from build123d import *

# Parameters (mm, degrees)
SKETCH1_W                         = 40
SKETCH1_H                         = 30
BOSS_EXTRUDE1_DEPTH               = 40
F_1_2_CLEARANCE_HOLE1_D           = 13.49248
F_1_2_CLEARANCE_HOLE1_CSINK_D     = 14.76248
F_1_2_CLEARANCE_HOLE1_CSINK_ANGLE = 100
CUT_EXTRUDE1_REACH                = 60.523
SKETCH4_R                         = 5
FILLET1_R                         = 5


with BuildPart() as part:
    # Sketch1 → Boss-Extrude1 (new body)
    with BuildSketch(Plane(origin=(0, 0, 0), x_dir=(1, 0, 0), z_dir=(0, 1, 0))):
        Rectangle(SKETCH1_W, SKETCH1_H)
    extrude(amount=BOSS_EXTRUDE1_DEPTH)

    # 1/2 Clearance Hole1 (through all)
    with Locations(Plane.XY.offset(15)):
        with Locations((0, 25)):
            CounterSinkHole(F_1_2_CLEARANCE_HOLE1_D / 2, F_1_2_CLEARANCE_HOLE1_CSINK_D / 2, counter_sink_angle=F_1_2_CLEARANCE_HOLE1_CSINK_ANGLE)

    # Sketch4 → Cut-Extrude1 (cut, up to next)
    with BuildSketch(Plane(origin=(20, 0, 0), x_dir=(0, 0, -1), z_dir=(1, 0, 0)), mode=Mode.PRIVATE) as cut_extrude1_sk1:
        with Locations((0, 10)):
            Circle(SKETCH4_R)
    cut_extrude1_tool1 = extrude(cut_extrude1_sk1.sketch, amount=-CUT_EXTRUDE1_REACH, mode=Mode.PRIVATE) & part.part
    add(cut_extrude1_tool1.solids().sort_by_distance((20, 10, 0))[0], mode=Mode.SUBTRACT)

    # Fillet1
    fillet1_edges = [part.edges().sort_by_distance(p)[0] for p in [
        (-20, 40, 0),
        (6.74624, 25, -15),
        (20, 40, 0),
        (-20, 0, 0),
        (20, 0, 0),
    ]]
    fillet(fillet1_edges, radius=FILLET1_R - 0.0001)  # a hair under: the kernel refuses the full size


solid = part.part
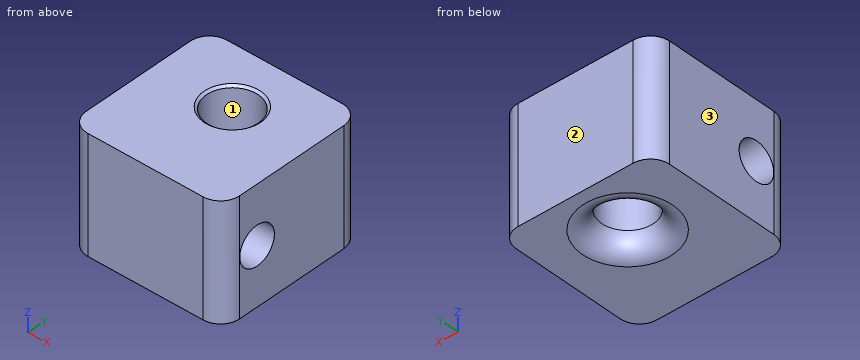
Check sheet for the modelled part. Datum: model origin and axes. Units: mm. Face numbers are marked on the shaded views. Round coordinates to 2 decimals unless told otherwise and drop trailing zeros. Loops run counter-clockwise (first coordinate to the right, second up) from the corner with the lowest first, then second, coordinate; pieces in that order, holes last.
1. Mould release check, pull along Y, two halves, no side actions. Record for the marked faces 1, 2 and 3: released by +Y, released by -Y, zero draft, split by the parting line, or undercut.
2. Gauge pin test, flat ends, axial feed: pin 1 Ø8 at (x, y) = (-3, 24) entering from -Z; pin 2 Ø12 at (x, y) = (0, 25) entering from +Z. Record the tip position at first contact, or that the pin passes through.
3. Sectioned sample at A-A on x = 0. Record the boundary of the cut face in (y, z).
4. Scan lines: probe 1 along Y at (x, z) = (-10, 0); probe 2 along X at (y, z) = (25, 7.75); probe 3 along Y at (x, z) = (1, -0.25). Record each from-to range of solid material in increasing order.
5. Sectioned sample at B-B on y = 25. Record the boundary of the cut face in (x, z), and give its area (3 significant figures).
6. Sectioned sample at C-C on z = 0. Give the number of separate pieces and of enclosed holes in the cut face, and give its area (3 significant figures).
7. Sectioned sample at D-D on z = -8. Record the boundary of the cut face in (x, y).
Recorded:
1. face 1: undercut
1. face 2: released by +Y
1. face 3: zero draft
2. pin 1: stops at z = -12
2. pin 2: passes through
3. outline: (0, -15) - (13.25, -15) arc R5 ccw to (18.25, -10) - (18.25, 14.47) - (17.62, 15) - (0, 15) - close; (31.75, -10) arc R5 ccw to (36.75, -15) - (40, -15) - (40, 15) - (32.38, 15) - (31.75, 14.47) - close; hole circle Ø10 at (10, 0)
4. probe 1: y = 0 to 5, 15 to 40
4. probe 2: x = -20 to -6.75, 6.75 to 20
4. probe 3: y = 0 to 5.01, 14.99 to 18.33, 31.67 to 40
5. outline: (-20, -15) - (-11.75, -15) arc R5 ccw to (-6.75, -10) - (-6.75, 14.47) - (-7.38, 15) - (-20, 15) - close; (6.75, -10) arc R5 ccw to (11.75, -15) - (20, -15) - (20, 15) - (7.38, 15) - (6.75, 14.47) - close
5. area: 784 mm2
6. separate pieces: 2
6. enclosed holes: 1
6. area: 1,040 mm2
7. outline: (-20, 5) arc R5 ccw to (-15, 0) - (15, 0) arc R5 ccw to (20, 5) - (20, 35) arc R5 ccw to (15, 40) - (-15, 40) arc R5 ccw to (-20, 35) - close; hole circle Ø13.49 at (0, 25)
